The model under review builds one solid part; all positions refer to its coordinate system, in mm. Face numbers are marked on the shaded views. A direction names the side the tool comes from. Give positions to 0.01 mm unless a question says otherwise; leave off trailing zeros. Loops run counter-clockwise (first coordinate to the right, second up) from the corner with the lowest first, then second, coordinate; pieces in that order, holes last. Notation, with made-up numbers: (27.25, 73.25) -> (75.25, 73.25) arc R33 cw to (75.25, 110.25) -> close; hole circle Ø7 at (50.25, 87.25). An arc over 180 degrees is marked (long way). Write each question's results on one line, items separated by ' | '. Start each with the question number.
Q1. Wall thickness on L1, parallel to Y at x = -0.4, z = -1.55; L2, parallel to Y at x = 1.05, z = 0.25; L3, parallel to X at y = 2.25, z = -0.7: over which ranges is each line inside the solid? List them lowest first. Write a range as [from, to].
Q2. Insertion check: pin 1 Ø2 at (x, y) = (1, 4) entering from -Z; pin 2 Ø1.1 at (x, z) = (0, -0.5) entering from +Y. Each pin has a flat end and moves straight along its axis. Give the tip position at first contact, or say it passes through.
Q3. We need section C-C (y = 6.25). Write out the cut boundary in (x, z).
Q4. Mouldability with a two-part tool opening along X and no side actions: class the marked faces 4, 5 and 6 as released by +X, released by -X, zero draft, split by the parting line, or undercut.
Q5. We need section D-D (y = 2.5). Write out the cut boundary in (x, z).
Q6. We need section A-A (z = 0). Write out the cut boundary in (x, y).
Q7. We need section B-B (x = 0.45). Write out the cut boundary in (y, z).
Q8. Machinability: for the marked faces 1, 2 and 3, which of the approach directions +Z, -Z, +X, -X, +Y, -Y give a long, thin tool a straight path to every point of the face, cutting with its end or side? Answer none if there is none.
Autodesk Inventor part; units mm, degrees
ref_plane "YZ Plane" through (0, 0, 0) normal (1, 0, 0) x (0, 1, 0)
ref_plane "XZ Plane" through (0, 0, 0) normal (0, 1, 0) x (-1, 0, 0)
ref_plane "XY Plane" through (0, 0, 0) normal (0, 0, 1) x (1, 0, 0)
sketch "Sketch1" plane through (0, 0, 0) normal (0, 1, 0) x (-1, 0, 0)
  circle A0 centre (0, 0) radius 1.25
  dimension "d0" = 2.5
extrude "Extrusion1" add sketch "Sketch1" along normal blind 6
sketch "Sketch2" plane through (0, 6, 0) normal (0, 1, 0) x (1, 0, 0)
  circle A0 centre (0, 0) radius 2
  dimension "d3" = 4
extrude "Extrusion2" add sketch "Sketch2" along normal blind 2
sketch "Sketch3" plane through (0, 8, 0) normal (0, 1, 0) x (1, 0, 0)
  circle A0 centre (0, 0) radius 1.25
  line L0 (0, 1.25) -> (1.0825, 0.625)
  line L1 (1.0825, 0.625) -> (1.0825, -0.625)
  line L2 (1.0825, -0.625) -> (0, -1.25)
  line L3 (0, -1.25) -> (-1.0825, -0.625)
  line L4 (-1.0825, -0.625) -> (-1.0825, 0.625)
  line L5 (-1.0825, 0.625) -> (0, 1.25)
extrude "Extrusion3" cut sketch "Sketch3" against normal blind 1.5 contours L1 L2 L3 L4 L5 L0
properties part number "M2.5_bolt"
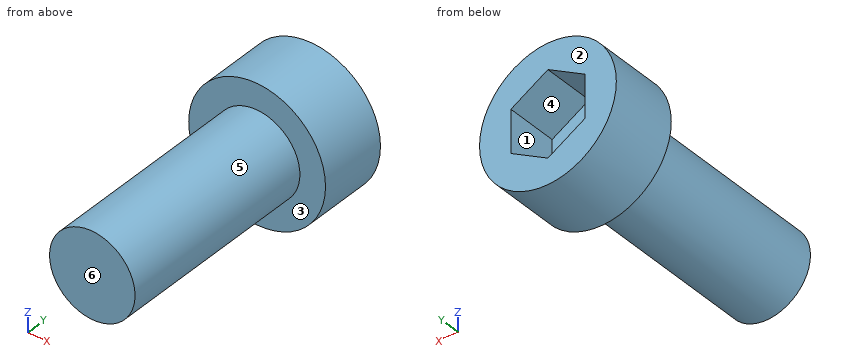
Output:
1) L1: [6, 8] | L2: [0, 6.5] | L3: [-1.04, 1.04]
2) pin 1: z = -1.25 | pin 2: y = 6.5
3) outline: circle Ø4 at (0, 0)
4) face 4: undercut | face 5: split by the parting line | face 6: zero draft
5) outline: circle Ø2.5 at (0, 0)
6) outline: (-2, 6) -> (-1.25, 6) -> (-1.25, 0) -> (1.25, 0) -> (1.25, 6) -> (2, 6) -> (2, 8) -> (1.08, 8) -> (1.08, 6.5) -> (-1.08, 6.5) -> (-1.08, 8) -> (-2, 8) -> close
7) outline: (0, -1.17) -> (6, -1.17) -> (6, -1.95) -> (8, -1.95) -> (8, -0.99) -> (6.5, -0.99) -> (6.5, 0.99) -> (8, 0.99) -> (8, 1.95) -> (6, 1.95) -> (6, 1.17) -> (0, 1.17) -> close
8) face 1: +Y | face 2: +Z, -Z, +X, -X, +Y | face 3: -Y
